```python
from build123d import *

# Parameters (mm, degrees)
SKETCH1_R              = 2.4
BOSS_EXTRUDE2_DEPTH    = 9
CUT_EXTRUDE2_START     = -12.485338913
CUT_EXTRUDE2_OUTLINE_R = 2.4
CUT_EXTRUDE2_DEPTH     = 8.07


# Read off the part's stored shape, not the designer's step: Cut-Extrude2
with BuildPart() as part:
    # Sketch1 → Boss-Extrude2 (new body)
    with BuildSketch(Plane(origin=(0, 0, 0), x_dir=(1, 0, 0), z_dir=(0, 1, 0))):
        with BuildLine():
            Line((-49.891335879, 12.485338913), (-67.821335879, 12.485338913))
            ThreePointArc((-67.821335879, 12.485338913), (-70.674511741, 11.303514775), (-71.856335879, 8.450338913))
            ThreePointArc((-71.856335879, 8.450338913), (-70.674511741, 5.597163051), (-67.821335879, 4.415338913))
            Line((-67.821335879, 4.415338913), (-49.891335879, 4.415338913))
            ThreePointArc((-49.891335879, 4.415338913), (-47.038160017, 5.597163051), (-45.856335879, 8.450338913))
            ThreePointArc((-45.856335879, 8.450338913), (-47.038160017, 11.303514775), (-49.891335879, 12.485338913))
        make_face()
        with Locations(Location((-67.821335879, 8.450338913, 0), (0, 0, 270))):
            Circle(SKETCH1_R, mode=Mode.SUBTRACT)
        with Locations(Location((-49.891335879, 8.450338913, 0), (0, 0, 270))):
            Circle(SKETCH1_R, mode=Mode.SUBTRACT)
    extrude(amount=BOSS_EXTRUDE2_DEPTH)

    # Cut-Extrude2 outline → Cut-Extrude2 (cut)
    with BuildSketch(Plane.XY.offset(CUT_EXTRUDE2_START)):
        with Locations((-58.856335879, 4.5)):
            Circle(CUT_EXTRUDE2_OUTLINE_R)
    extrude(amount=CUT_EXTRUDE2_DEPTH, mode=Mode.SUBTRACT)


solid = part.part
```
Input: part model. Units: mm. Frame: model coordinates. Round coordinates to 2 decimals unless told otherwise and drop trailing zeros. Loops run counter-clockwise (first coordinate to the right, second up) from the corner with the lowest first, then second, coordinate; pieces in that order, holes last. Notation, with made-up numbers: (21.25, 53.25) - (29.25, 53.25) arc R36 cw to (29.25, 91.25) - close; hole circle Ø11 at (-3, 22.25). An arc over 180 degrees is marked (long way). One line per item, written item: value. Start each with the question number.
(1) Section B-B, the plane z = -8. Return loops of the section in (x, y).
(2) Contact query for flat-ended pins moving along their axis: P1, Ø4, axis at x = -55.5, z = -10.5, coming from the -Y side; P2, Ø2, axis at y = 6.5, z = -11, coming from the -X side. Output: stop coordinate, or through.
(3) Section A-A, the plane y = 4.5. Return loops of the section in (x, z) (3 decimals).
(4) Ray query, line 1 (X direction, y = 0.5, z = -8); line 2 (X direction, y = 8.25, z = -7.25); line 3 (Z direction, x = -68, y = 7.25). Return the intervals inside material, ascending. Write a range as [from, to].
(5) Section C-C, the plane z = -5. Return loops of the section in (x, y).
(6) Section D-D, the plane y = 3. Return loops of the section in (x, z) (3 decimals), plus the area to 3 significant figures.
(7) Draft query along X for faces 1 (the flat face through (-59, 0, -9)), 2 (the cylindrical face through (-69.95, 4.44, -7.34)). Return one class per face: +X half, -X half, draft (parallel to the pull), parting line (faces both ways), or undercut.
Results below:
1. outline: (-71.83, 0) - (-70.18, 0) - (-70.18, 9) - (-71.83, 9) - close; (-65.46, 0) - (-52.25, 0) - (-52.25, 9) - (-65.46, 9) - close; (-47.53, 0) - (-45.88, 0) - (-45.88, 9) - (-47.53, 9) - close; hole circle Ø4.8 at (-58.86, 4.5)
2. P1: y = 0
2. P2: x = -71.55
3. outline: (-67.821, -12.485) - (-61.256, -12.485) - (-61.256, -4.415) - (-67.821, -4.415) arc R4.035 ccw to start; (-56.456, -12.485) - (-49.891, -12.485) arc R4.035 ccw to (-49.891, -4.415) - (-56.456, -4.415) - close; hole circle Ø4.8 at (-67.821, -8.45); hole circle Ø4.8 at (-49.891, -8.45)
4. line 1: [-71.83, -70.18], [-65.46, -52.25], [-47.53, -45.88]
4. line 2: [-71.67, -69.9], [-65.74, -51.97], [-47.81, -46.04]
4. line 3: [-12.48, -10.84], [-6.06, -4.42]
5. outline: (-69.91, 0) - (-47.8, 0) - (-47.8, 9) - (-69.91, 9) - close; hole circle Ø4.8 at (-58.86, 4.5)
6. outline: (-67.821, -12.485) - (-60.73, -12.485) - (-60.73, -4.415) - (-67.821, -4.415) arc R4.035 ccw to start; (-56.983, -12.485) - (-49.891, -12.485) arc R4.035 ccw to (-49.891, -4.415) - (-56.983, -4.415) - close; hole circle Ø4.8 at (-67.821, -8.45); hole circle Ø4.8 at (-49.891, -8.45)
6. area: 129 mm^2
7. face 1: draft
7. face 2: undercut
